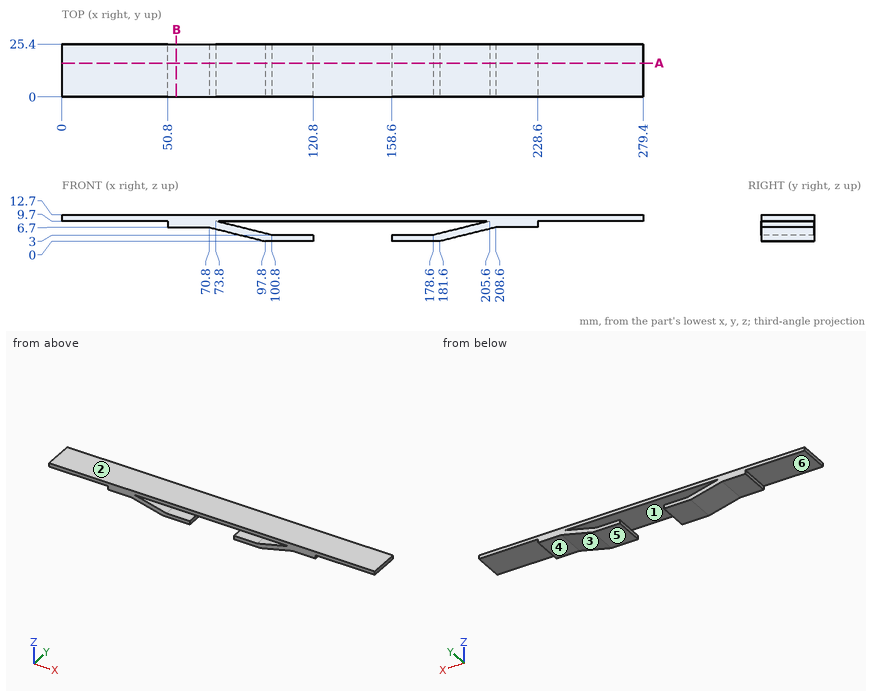
Design review of the part shown in the three views and the two pictorial views. Dimensions are in mm from the part's minimum x, y and z. A direction names the side the tool comes from. Round coordinates to 2 decimals unless told otherwise and drop trailing zeros. Loops run counter-clockwise (first coordinate to the right, second up) from the corner with the lowest first, then second, coordinate; pieces in that order, holes last. Notation, with made-up numbers: (-12.5, 56.25) - (-1.5, 56.25) arc R23 cw to (-1.5, 94.25) - close; hole circle Ø1 at (-6, 69.25). An arc over 180 degrees is marked (long way). One line per item, written item: value. Start each with the question number.
Item 1: Take a section at B-B (x = 55). Give the boundary of the cut face in (y, z).
Item 2: Take a section at A-A (y = 16.25). Give the boundary of the cut face in (x, z).
Item 3: For the marked faces 4, 5 and 6, list the 3-axis set-ups (+Z, -Z, +X, -X, +Y, -Y) from which the entire face can be reached by the end or side of a thin tool; tool diameter is ignored.
Item 4: The part is to be moulded in two halves that separate along Z. For the marked faces 1, 2 and 3, say which applies: +Z half, -Z half, draft (parallel to the pull), parting line (faces both ways), or undercut.
Item 5: For L1, parallel to Z at x = 109, y = 17.75; L2, parallel to Z at x = 133, y = 22.5; L3, parallel to Z at x = 212, y = 17.5, list the stretches that pass through material, from the lowest coordinate up.
Item 6: Clearance check with flat-ended pins moving along their axes: pin 1 Ø1.5 at (y, z) = (14, 8.5) entering from +X; pin 2 Ø7.5 at (x, y) = (30.5, 12.5) entering from -Z; pin 3 Ø10 at (x, y) = (218, 11) entering from -Z. State where each tip first meets the part, or that it passes through.
Answer below:
1. outline: (0, 6.7) - (25.4, 6.7) - (25.4, 12.7) - (0, 12.7) - close
2. outline: (0, 9.7) - (50.8, 9.7) - (50.8, 6.7) - (70.8, 6.7) - (97.8, 0) - (120.8, 0) - (120.8, 3) - (100.8, 3) - (73.8, 9.7) - (205.6, 9.7) - (178.6, 3) - (158.6, 3) - (158.6, 0) - (181.6, 0) - (208.6, 6.7) - (228.6, 6.7) - (228.6, 9.7) - (279.4, 9.7) - (279.4, 12.7) - (0, 12.7) - close
3. face 4: -Z, +X, +Y, -Y
3. face 5: -Z, +X, -X, +Y, -Y
3. face 6: -Z, -X, +Y, -Y
4. face 1: undercut
4. face 2: +Z half
4. face 3: -Z half
5. L1: z = 0 to 3, 9.7 to 12.7
5. L2: z = 9.7 to 12.7
5. L3: z = 6.7 to 12.7
6. pin 1: stops at x = 228.6
6. pin 2: stops at z = 9.7
6. pin 3: stops at z = 6.7
